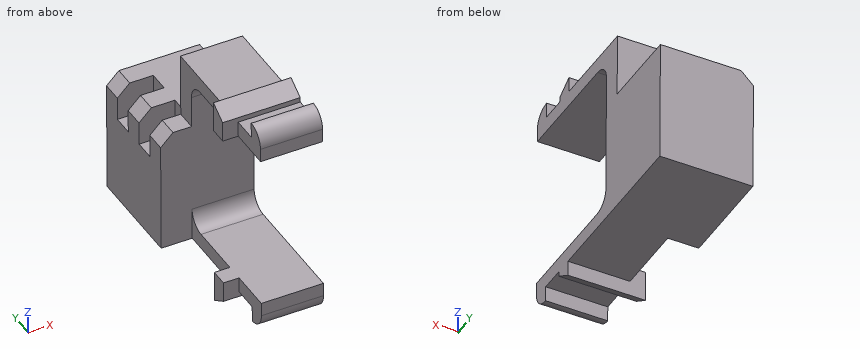
```python
from build123d import *

# Parameters (mm, degrees)
PAD017_DEPTH              = 5
PAD020_DEPTH              = 6.25
SKETCH038_W               = 10
SKETCH038_H               = 1.65
PAD021_DEPTH              = 5
SKETCH085_W               = 10
SKETCH085_H               = 1.65
PAD054_DEPTH              = 7.5
SKETCH083_W               = 7.1
SKETCH083_H               = 1.65
PAD055_DEPTH              = 7.5
SKETCH082_W               = 10
SKETCH082_H               = 1.65
PAD056_DEPTH              = 4.6
SKETCH084_W               = 10
SKETCH084_H               = 1.65
PAD057_DEPTH              = 7.5
LINEARPATTERN019_COUNT    = 2
LINEARPATTERN019_PITCH    = 3.3
CHAMFER009_SIZE           = 1
MIRROR008_PLACEMENT_ANGLE = 90


with BuildPart() as obj1:
    # Sketch034 → Pad017 (new body)
    with BuildSketch(Plane.XY):
        with BuildLine():
            Line((-1.35, -1.8), (-1.35, 6))
            ThreePointArc((0, 7.35), (-0.954594, 6.954594), (-1.35, 6))
            Line((0, 9), (0, 7.35))
            Line((-2.6, 9), (0, 9))
            Line((-2.6, -1.8), (-2.6, 9))
            Line((-3.85, -1.8), (-2.6, -1.8))
            ThreePointArc((-3.85, -1.8), (-3.439949, -2.789949), (-2.45, -3.2))
            Line((-1.35, -3.2), (-2.45, -3.2))
            Line((-1.35, -1.8), (-1.35, -3.2))
        make_face()
    extrude(amount=PAD017_DEPTH)

    # Sketch037 → Pad020 (join)
    with BuildSketch(Plane.XY):
        Polygon((-1.35, 0.2), (-1.35, 1.6), (-2.6, 1.6), (-3.85, 1.6), (-3, 0.2), (-2.6, 0.2), align=None)
    extrude(amount=PAD020_DEPTH)


with BuildPart() as body029:
    # Mirror002: instance of _obj1
    add(obj1.part.mirror(Plane(origin=(5, 0, 0), x_dir=(0, 1, 0), z_dir=(-1, 0, 0))))

    # Fusion002: union _obj1
    add(obj1.part)


with BuildPart() as body029_1:
    # Clone003 placement: moved
    add(body029.part.moved(Location((-5, 0, 0))))

    # Sketch038 → Pad021 (new body)
    with BuildSketch(Plane.XY):
        with Locations((0, 8.175)):
            Rectangle(SKETCH038_W, SKETCH038_H)
    extrude(amount=PAD021_DEPTH)

    # Sketch085 → Pad054 (new body)
    with BuildSketch(Plane.XY):
        with Locations((2.6, 8.175)):
            Rectangle(SKETCH085_W, SKETCH085_H)
    extrude(amount=PAD054_DEPTH)

    # Sketch083 → Pad055 (join)
    with BuildSketch(Plane.XY):
        with Locations((4.05, 9.825)):
            Rectangle(SKETCH083_W, SKETCH083_H)
    pad055 = extrude(amount=PAD055_DEPTH)

    # Sketch082 → Pad056 (join)
    with BuildSketch(Plane.XY):
        with Locations((2.6, 9.825)):
            Rectangle(SKETCH082_W, SKETCH082_H)
    pad056 = extrude(amount=PAD056_DEPTH)

    # Sketch084 → Pad057 (join)
    with BuildSketch(Plane.XY):
        with Locations((2.6, 11.475)):
            Rectangle(SKETCH084_W, SKETCH084_H)
    pad057 = extrude(amount=PAD057_DEPTH)

    # LinearPattern019: Pad057, Pad056, Pad055 ×2
    with Locations(*[(0, i * LINEARPATTERN019_PITCH, 0) for i in range(1, LINEARPATTERN019_COUNT)]):
        add(pad057)
        add(pad056)
        add(pad055)

    # Chamfer009
    chamfer009_edges = [body029_1.edges().sort_by_distance(p)[0] for p in [
        (-2.4, 8.175, 7.5),
        (-2.4, 11.475, 7.5),
        (-2.4, 14.775, 7.5),
    ]]
    chamfer(chamfer009_edges, length=CHAMFER009_SIZE)


with BuildPart() as mirror008:
    # Mirror008: instance of Body029
    add(body029_1.part.mirror(Plane(origin=(-13.185052, -8.707698, 3.680996), x_dir=(-0.004692, 0.999989, 0), z_dir=(-0.999989, -0.004692, -1e-06))))


with BuildPart() as mirror008_1:
    # Mirror008 placement: moved
    add(mirror008.part.moved(Location((2.5, 0, 34.15))).rotate(Axis((2.5, 0, 34.15), (0, -1, 0)), MIRROR008_PLACEMENT_ANGLE))


solid = mirror008_1.part
```
Design review of the part built by this model. Coordinates are the model's own, in mm. Give positions to 0.01 mm unless a question says otherwise; leave off trailing zeros. Loops run counter-clockwise (first coordinate to the right, second up) from the corner with the lowest first, then second, coordinate; pieces in that order, holes last. Notation, with made-up numbers: M -1.5,69.25 L 11.5,69.25 A19 cw 11.5,73.25 Z; hole C 78,62 d2. An arc over 180 degrees is marked long. Return JSON: item names as keys, results as strings. Group by question number.
Item 1: Insertion check: pin 1 Ø0.8 at (y, z) = (5, 1.5) entering from -X; pin 2 Ø1 at (x, y) = (-3.5, 12) entering from +Z; pin 3 Ø1.3 at (y, z) = (13, 9) entering from -X; pin 4 Ø1.6 at (y, z) = (5.5, 12.5) entering from -X. Each pin has a flat end and moves straight along its axis. Give the tip position at first contact, or say it passes through.
Item 2: We need section C-C (y = 13.5). Give the boundary of the cut face in (x, z).
Item 3: We need section D-D (z = 8.5). Give the boundary of the cut face in (x, y).
Item 4: We need section B-B (z = 14.5). Give the boundary of the cut face in (x, y), and give its area (3 significant figures).
Item 5: For probe 1 along Y at (x, z) = (1.5, 9); probe 2 along Z at (x, y) = (-2.75, 0.75); probe 3 along Y at (x, z) = (2.25, 0.25), list the stretches that pass through material, from the lowest coordinate up.
Item 6: We need section A-A (y = 0.5). Give the boundary of the cut face in (x, z), and give its area (3 significant figures).
Output:
{
 "1": {"pin 1": "stops at x = -2.5", "pin 2": "stops at z = 9.99", "pin 3": "stops at x = -2.1", "pin 4": "passes through"},
 "2": {"outline": "M -5,-0.03 L 2.5,-0.03 L 2.5,9.97 L -2.1,9.97 L -2.1,7.07 L -5,7.07 Z"},
 "3": {"outline": "M -5,7.23 L 2.5,7.23 L 2.5,15.48 L -5,15.48 L -5,13.83 L -2.1,13.83 L -2.1,12.18 L -5,12.18 L -5,10.53 L -2.1,10.53 L -2.1,8.88 L -5,8.88 Z"},
 "4": {"outline": "M -3.75,0.14 L -2.5,0.14 L -2.5,-3.26 L 2.5,-3.26 L 2.5,8.94 L -2.5,8.94 L -2.5,1.54 L -3.75,1.54 Z", "area": "62.8 mm^2"},
 "5": {"probe 1": "y = 7.24 to 15.49", "probe 2": "z = -0.77 to 1.34, 14.04 to 16.05", "probe 3": "y = -3.39 to 15.41"},
 "6": {"outline": "M -3.75,-0.61 L 2.5,-0.61 L 2.5,1.34 L -3.75,1.34 Z; M -3.75,14.04 L 2.5,14.04 L 2.5,15.9 L -3.75,15.9 Z", "area": "23.8 mm^2"}
}
